```python
from build123d import *

# Parameters (mm, degrees)
F0_W     = 80
F0_H     = 80
F1_DEPTH = 25
F3_DEPTH = 80
F5_DEPTH = 80


with BuildPart() as f1:
    # F0 (on Front) → F1 (new body)
    with BuildSketch(Plane.XZ):
        with Locations((0.42491, 6.112343)):
            Rectangle(F0_W, F0_H)
    extrude(amount=-F1_DEPTH)

    # F2 (on face) → F3 (cut)
    with BuildSketch(Plane(origin=(0, 0, -33.887657), x_dir=(1, 0, 0), z_dir=(0, 0, -1))):
        Polygon((-5.96826, 0), (-10, -10), (10, -10), (6.775631, 0), align=None)
    extrude(amount=-F3_DEPTH, mode=Mode.SUBTRACT)

    # F4 (on face) → F5 (cut)
    with BuildSketch(Plane(origin=(-39.57509, 0, 0), x_dir=(0, -1, 0), z_dir=(-1, 0, 0))):
        Polygon((-10, 16.112343), (-10, 6.112343), (-10, -3.887657), (0, -0.294908), (0, 12.498255), align=None)
    extrude(amount=-F5_DEPTH, mode=Mode.SUBTRACT)


solid = f1.part
```
Geometry: final body of the model. Coordinates: model frame, mm. A direction names the side the tool comes from. Round coordinates to 2 decimals unless told otherwise and drop trailing zeros. Order: outer loops, then holes, each group sorted by start corner. A loop starts at its lowest first (then second) coordinate and runs counter-clockwise, first axis right, second up. Notation, with made-up numbers: (77.5, 62.25) -> (129.5, 62.25) arc R15 ccw to (129.5, 85.25) -> close; hole circle Ø4 at (37, 62). An arc over 180 degrees is marked (long way). Use CSV: the item, a comma, the result in double quotes. Start each with the question number.
1) Section D-D (z = -16). Return the cut outline in (x, y), and give its area (3 significant figures).
2) Material intervals for line 1 along Z through (x, y) = (-28.5, 1.5); line 2 along X through (y, z) = (5.25, -21.5); line 3 along Y through (x, z) = (-8, -8.5), sorted ascending. Write a range as from..to.
3) Set-up query: faces 1 (the face through (-7.956, 4.93, -17.326)), 2 (the face through (0, 12, -33.888)), 3 (the face through (0, 10, 7)), 4 (the face through (23.365, 5.07, -2.116)). Return all of +Z, -Z, +X, -X, +Y, -Y with unobstructed straight access to the full face (end or side cutting, diameter ignored); none if empty.
4) Section B-B (z = 15). Return the cut outline in (x, y), and give its area (3 significant figures).
5) Section C-C (y = 3.75). Return the cut outline in (x, z).
6) First-contact query: pin 1 Ø6 at (x, z) = (23, 9) entering from -Y. Flat tip, straight axial feed; report the tip coordinate or a pass-through.
7) Section A-A (x = 13). Return the cut outline in (y, z).
8) Draft query along Z for faces 5 (the face through (0, 12, 46.112)), 6 (the face through (-23, 0, -17)), 7 (the face through (-23.01, 4.93, 14.28)). Return one class per face: +Z half, -Z half, draft (parallel to the pull), parting line (faces both ways), or undercut.
Returned:
1,outline,"(-39.58, 0) -> (-5.97, 0) -> (-10, 10) -> (10, 10) -> (6.78, 0) -> (40.42, 0) -> (40.42, 25) -> (-39.58, 25) -> close"
1,area,"1,840 mm²"
2,line 1,"z = -33.89..-0.83, 13.04..46.11"
2,line 2,"x = -39.58..-8.08, 8.47..40.42"
2,line 3,"y = 0..5.04, 10..25"
3,face 1,"+Z, -Z"
3,face 2,"-Z, +X, -X, +Y, -Y"
3,face 3,"none"
3,face 4,"+X, -X"
4,outline,"(-39.58, 0) -> (-5.97, 0) -> (-8.76, 6.92) -> (-39.58, 6.92) -> close; (-39.58, 10) -> (40.42, 10) -> (40.42, 25) -> (-39.58, 25) -> close; (6.78, 0) -> (40.42, 0) -> (40.42, 6.92) -> (9.01, 6.92) -> close"
4,area,"1,650 mm²"
5,outline,"(-39.58, -33.89) -> (-7.48, -33.89) -> (-7.48, -1.64) -> (-39.58, -1.64) -> close; (-39.58, 13.85) -> (-7.48, 13.85) -> (-7.48, 46.11) -> (-39.58, 46.11) -> close; (7.98, -33.89) -> (40.42, -33.89) -> (40.42, -1.64) -> (7.98, -1.64) -> close; (7.98, 13.85) -> (40.42, 13.85) -> (40.42, 46.11) -> (7.98, 46.11) -> close"
6,pin 1,"stops at y = 10"
7,outline,"(0, -33.89) -> (25, -33.89) -> (25, 46.11) -> (0, 46.11) -> (0, 12.5) -> (10, 16.11) -> (10, -3.89) -> (0, -0.29) -> close"
8,face 5,"+Z half"
8,face 6,"draft"
8,face 7,"undercut"
